Could you check a few things on this model? Use its own coordinates, in mm. Give positions to 0.01 mm unless a question says otherwise; leave off trailing zeros. Write each loop counter-clockwise with the first axis right and the second up, starting at its lowest first coordinate (ties: lowest second). Pieces come first, ordered by that corner, then holes. Notation, with made-up numbers: (73.25, 70) -> (96.25, 70) arc R26 cw to (96.25, 106) -> close; hole circle Ø11 at (18, 40). An arc over 180 degrees is marked (long way). One line per question, with ' | ' between items.
from build123d import *

# Parameters (mm, degrees)
F0_R     = 10.16
F0_R_2   = 4.318
F1_DEPTH = 7.9375
F2_R     = 1.778
F3_DEPTH = 25.4
F4_SIZE  = 0.4


with BuildPart() as f1:
    # F0 (on Top) → F1 (new body)
    with BuildSketch(Plane.XY):
        Circle(F0_R)
        Circle(F0_R_2, mode=Mode.SUBTRACT)
    extrude(amount=F1_DEPTH)

    # F2 (on Front) → F3 (cut)
    with BuildSketch(Plane.XZ):
        with Locations((0, 4.1275)):
            Circle(F2_R)
    extrude(amount=-F3_DEPTH, mode=Mode.SUBTRACT)

    # F4
    f4_edges = [f1.edges().sort_by_distance(p)[0] for p in [
        (-10.16, 0, 0),
        (-10.16, 0, 7.9375),
    ]]
    chamfer(f4_edges, length=F4_SIZE)


solid = f1.part
Q1. Imagine slicing it at A-A on x = 0. Please give me the cut outline in (y, z), and give its area (3 significant figures).
Answer below:
outline: (-10.16, 0.4) -> (-9.76, 0) -> (-4.32, 0) -> (-4.32, 7.94) -> (-9.76, 7.94) -> (-10.16, 7.54) -> close; (4.32, 0) -> (9.76, 0) -> (10.16, 0.4) -> (10.16, 2.35) -> (4.32, 2.35) -> close; (4.32, 5.91) -> (10.16, 5.91) -> (10.16, 7.54) -> (9.76, 7.94) -> (4.32, 7.94) -> close | area: 71.6 mm^2
Q2. If we mould it in two halves opening along X, with no side actions, what happens to faces 1 (the cylindrical face through (-0.23, 7.01, 5.89)), 2 (the cylindrical face through (-2.2, -9.92, 3.92)), 3 (the flat face through (2, -4, 0)), 4 (the cylindrical face through (-0.936, -4.215, 3.913))? For each: +X half, -X half, draft (parallel to the pull), parting line (faces both ways), or undercut.
Answer below:
face 1: undercut | face 2: parting line | face 3: draft | face 4: undercut
Q3. Imagine slicing it at B-B on y = 0. Please give me the cut outline in (x, z), and give its area (3 significant figures).
Answer below:
outline: (-10.16, 0.4) -> (-9.76, 0) -> (-4.32, 0) -> (-4.32, 7.94) -> (-9.76, 7.94) -> (-10.16, 7.54) -> close; (4.32, 0) -> (9.76, 0) -> (10.16, 0.4) -> (10.16, 7.54) -> (9.76, 7.94) -> (4.32, 7.94) -> close | area: 92.4 mm^2
Q4. If I drill on line 1 along Y through (x, z) = (0, 2.25); line 2 along Z through (x, y) = (0, 7); line 3 along Y through (x, z) = (0, 5), over which ranges is the centre line in solid material (lowest first)?
Answer below:
line 1: y = -10.16 to -4.32, 4.32 to 10.16 | line 2: z = 0 to 2.35, 5.91 to 7.94 | line 3: y = -10.16 to -4.32
Q5. Imagine slicing it at C-C on z = 7.25. Please give me the cut outline in (x, y).
Answer below:
outline: circle Ø20.32 at (0, 0); hole circle Ø8.64 at (0, 0)
Q6. Will these pins go through, and if not, where does the flat tip stop? pin 1 (2 mm diameter, centred on y = -0.5, z = 2.5, fed in from +X); pin 2 (4 mm diameter, centred on y = 6, z = 6.5, fed in from -X); pin 3 (3 mm diameter, centred on x = -5.5, z = 3, fed in from +Y); pin 4 (1.5 mm diameter, centred on y = 5.5, z = 4, fed in from -X).
Answer below:
pin 1: stops at x = 10.16 | pin 2: stops at x = -9.34 | pin 3: stops at y = 9.34 | pin 4: stops at x = -8.98
Q7. Imagine slicing it at D-D on z = 3.25. Please give me the cut outline in (x, y), and give its area (3 significant figures).
Answer below:
outline: (-1.55, 4.03) -> (-1.55, 10.04) arc R10.16 ccw (long way) to (1.55, 10.04) -> (1.55, 4.03) arc R4.32 cw (long way) to start | area: 247 mm^2
